```python
from build123d import *

# Parameters (mm, degrees)
F1_DEPTH      = 10
F3_DEPTH      = 10
F4_DEPTH      = 9
F5_DEPTH      = 9
F6_SIZE2      = 2.49999
F6_SIZE       = 1.49999
F7_R          = 0.8
F8_R          = 0.8
F9_R          = 0.8
F10_T1_DEPTH  = 10
F10_T4_ANGLE  = 88.2100893918
F10_T6_ANGLE  = 88.2100893918
F10_T8_ANGLE  = 88.2100893918
F10_T10_ANGLE = 88.2100893918


# Not quite as in the source:
# - a fillet or chamfer that OpenCascade refuses, or shapes differently, is made with other operations: its cross-section is extruded or revolved along the edge and cut away or added
# - a fillet or chamfer is up to 0.001 mm smaller than in the source, because OpenCascade refuses the exact size


with BuildPart() as f1:
    # F0 (on Top) → F1 (new body)
    with BuildSketch(Plane.XY):
        Polygon((27.5, 0), (-27.5, 0), (-28, 16), (-30.9985362283, 15.9062957429), (-30.4077144863, -3), (30.4077144863, -3), (30.9985362283, 15.9062957429), (28, 16), align=None)
        Polygon((-30.9985362283, 15.9062957429), (-28, 16), (-24.0019516957, 16.1249390095), (-24.0956559528, 19.1234752378), (-35.0902887897, 18.7798929616), (-34.9965845326, 15.7813567334), align=None)
        Polygon((24.0019516957, 16.1249390095), (28, 16), (30.9985362283, 15.9062957429), (34.9965845326, 15.7813567334), (34.9965845326, 18.7813567334), (24.0019516957, 19.1249390095), align=None)
    extrude(amount=F1_DEPTH)

    # F2 (on Right) → F3 (join, symmetric)
    with BuildSketch(Plane.YZ):
        Polygon((-3, 16), (-3, 10), (-0.5, 10), (-0.5, 20), (-3, 20), align=None)
    extrude(amount=F3_DEPTH, both=True)

    # F2 (on Right) → F4 (join, symmetric)
    with BuildSketch(Plane.YZ):
        Polygon((-3, 1.5), (-3, 10), (-3, 16), (-5, 16), (-5, 1.5), align=None)
    extrude(amount=F4_DEPTH, both=True)

    # F2 (on Right) → F5 (join, symmetric)
    with BuildSketch(Plane.YZ):
        Polygon((-5, 0), (-5, 1.5), (-5, 16), (-5, 18), (-7.5, 18), (-7.5, 0), align=None)
    extrude(amount=F5_DEPTH, both=True)

    # F6 (size 1.5 and 2.5 in the source; OpenCascade refuses exactly that, so slightly less here)
    f6_edges = [f1.edges().sort_by_distance(p)[0] for p in [
        (0, -7.5, 18),
        (-9, -7.5, 9),
        (9, -7.5, 9),
    ]]
    f6_side = f1.faces().sort_by_distance((0, -7.5, 9))[0]
    chamfer(f6_edges, length=F6_SIZE, length2=F6_SIZE2, reference=f6_side)

    # F7
    f7_edges = [f1.edges().sort_by_distance(p)[0] for p in [
        (27.75, 8, 0),
        (0, 0, 0),
        (-27.75, 8, 0),
        (-26.000976, 16.06247, 0),
        (-24.048804, 17.624207, 0),
        (-29.592972, 18.951684, 0),
        (-35.043437, 17.280625, 0),
        (-32.99756, 15.843826, 0),
        (-30.703125, 6.453148, 0),
        (0, -3, 0),
        (30.703125, 6.453148, 0),
        (32.99756, 15.843826, 0),
        (34.996585, 17.281357, 0),
        (29.499268, 18.953148, 0),
        (24.001952, 17.624939, 0),
        (26.000976, 16.06247, 0),
    ]]
    fillet(f7_edges, radius=F7_R)

    # F8
    f8_edges = [f1.edges().sort_by_distance(p)[0] for p in [
        (-29.592972, 18.951684, 10),
        (-35.043437, 17.280625, 10),
        (-32.99756, 15.843826, 10),
        (-26.000976, 16.06247, 10),
        (-24.048804, 17.624207, 10),
        (-27.75, 8, 10),
        (-30.703125, 6.453148, 10),
        (-20.203857, -3, 10),
        (20.203857, -3, 10),
        (30.703125, 6.453148, 10),
        (32.99756, 15.843826, 10),
        (34.996585, 17.281357, 10),
        (29.499268, 18.953148, 10),
        (24.001952, 17.624939, 10),
        (26.000976, 16.06247, 10),
        (27.75, 8, 10),
    ]]
    fillet(f8_edges, radius=F8_R)

    # F9
    f9_edges = [f1.edges().sort_by_distance(p)[0] for p in [
        (0, -0.5, 20),
        (-10, -0.5, 15),
        (10, -0.5, 15),
        (10, -1.75, 20),
        (-10, -1.75, 20),
    ]]
    fillet(f9_edges, radius=F9_R)

    # F10: fillet of radius 2 on 2 edges, made by hand

    # F10_s2 → F10_t1 (cut)
    with BuildSketch(Plane.XY):
        with BuildLine():
            ThreePointArc((-28.4692381621, -3), (-29.861190207, -2.4361300445), (-30.4682623143, -1.0624695048))
            Line((-30.4682623143, -1.0624695048), (-30.4077144863, -3))
            Line((-30.4077144863, -3), (-28.4692381621, -3))
        make_face()
        with BuildLine():
            ThreePointArc((28.4692381621, -3), (29.861190207, -2.4361300445), (30.4682623143, -1.0624695048))
            Line((30.4682623143, -1.0624695048), (30.4077144863, -3))
            Line((30.4077144863, -3), (28.4692381621, -3))
        make_face()
    extrude(amount=F10_T1_DEPTH, mode=Mode.SUBTRACT)

    # F10_s3 → F10_t4 (revolve, cut)
    with BuildSketch(Plane(origin=(-0.0034446457, -0.1102286623, 0), x_dir=(0, 0, 1), z_dir=(0.0312347524, 0.9995120761, 0))):
        with BuildLine():
            ThreePointArc((0, 29.6865820924), (0.2343145751, 30.2522675173), (0.8, 30.4865820924))
            Line((0.8, 30.4865820924), (0, 30.4865820924))
            Line((0, 30.4865820924), (0, 29.6865820924))
        make_face()
    revolve(axis=Axis((28.4692381621, -1, 0), (0, 0, -1)), revolution_arc=F10_T4_ANGLE, mode=Mode.SUBTRACT)

    # F10_s5 → F10_t6 (revolve, cut)
    with BuildSketch(Plane.YZ.offset(28.4692381621)):
        with BuildLine():
            ThreePointArc((-2.2, 10), (-2.7656854249, 9.7656854249), (-3, 9.2))
            Line((-3, 9.2), (-3, 10))
            Line((-3, 10), (-2.2, 10))
        make_face()
    revolve(axis=Axis((28.4692381621, -1, 10), (0, 0, 1)), revolution_arc=F10_T6_ANGLE, mode=Mode.SUBTRACT)

    # F10_s7 → F10_t8 (revolve, cut)
    with BuildSketch(Plane.YZ.offset(-28.4692381621)):
        with BuildLine():
            ThreePointArc((-2.2, 0), (-2.7656854249, 0.2343145751), (-3, 0.8))
            Line((-3, 0.8), (-3, 0))
            Line((-3, 0), (-2.2, 0))
        make_face()
    revolve(axis=Axis((-28.4692381621, -1, 0), (0, 0, -1)), revolution_arc=F10_T8_ANGLE, mode=Mode.SUBTRACT)

    # F10_s9 → F10_t10 (revolve, cut)
    with BuildSketch(Plane(origin=(0.0034446457, -0.1102286623, 0), x_dir=(0, 0, 1), z_dir=(-0.0312347524, 0.9995120761, 0))):
        with BuildLine():
            ThreePointArc((10, -29.6865820924), (9.7656854249, -30.2522675173), (9.2, -30.4865820924))
            Line((9.2, -30.4865820924), (10, -30.4865820924))
            Line((10, -30.4865820924), (10, -29.6865820924))
        make_face()
    revolve(axis=Axis((-28.4692381621, -1, 10), (0, 0, 1)), revolution_arc=F10_T10_ANGLE, mode=Mode.SUBTRACT)


solid = f1.part
```
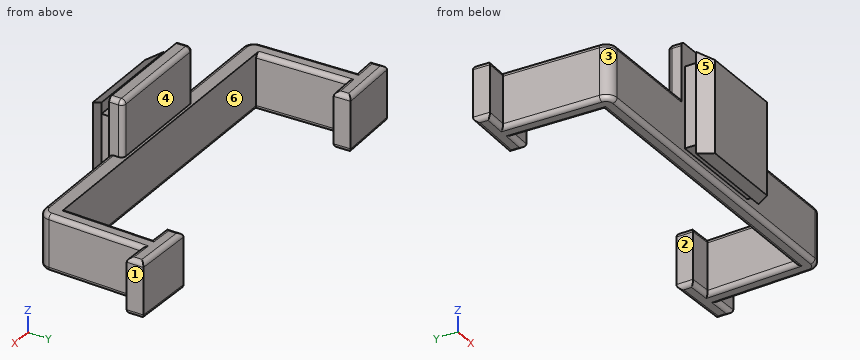
Can you work these out from the model? Positions are in its coordinate system, mm. Face numbers are marked on the shaded views. A direction names the side the tool comes from. Round coordinates to 2 decimals unless told otherwise and drop trailing zeros. Loops run counter-clockwise (first coordinate to the right, second up) from the corner with the lowest first, then second, coordinate; pieces in that order, holes last. Notation, with made-up numbers: M 73.25,64.5 L 117.25,64.5 A26 cw 117.25,78.5 Z; hole C 76,25.5 d1. An arc over 180 degrees is marked long. Answer as a JSON object with one key per item and string values. Group by question number.
Q1. We'd pull the mould along X, two halves only. Please class the marked faces 1, 2 and 3: +X half, -X half, draft (parallel to the pull), parting line (faces both ways), or undercut.
Q2. Imagine slicing it at B-B, the plane z = 11.75. Please give me the cut outline in (x, y), then the cut area to 3 significant figures.
Q3. Will these pins go through, and if not, where does the flat tip stop? pin 1 (1.9 mm diameter, centred on y = -1.5, z = 12, fed in from -X); pin 2 (12 mm diameter, centred on y = 2, z = 15, fed in from +X); pin 3 (1 mm diameter, centred on y = 6.5, z = 8, fed in from -X); pin 4 (3 mm diameter, centred on y = 7.5, z = 12.5, fed in from +X).
Q4. Imagine slicing it at A-A, the plane x = 22.5. Please give me the cut outline in (y, z), then the cut area to 3 significant figures.
Q5. Imagine slicing it at C-C, the plane z = 3.25. Please give me the cut outline in (x, y), then the cut area to 3 significant figures.
Q6. Please list where these lines run through material, in increasing order: L1, parallel to Z at x = -30, y = 13.75; L2, parallel to X at y = 14.25, z = 3; L3, parallel to Y at x = 6.5, z = 6.75.
Q7. On a 3-axis mill with a long thin cutter (end or side, diameter ignored), from which of +Z, -Z, +X, -X, +Y, -Y can I reach the whole of each face in a straight line? I mean the marked faces 4, 5 and 6. Say none if no direction works.
Findings:
{
 "1": {"face 1": "+X half", "face 2": "undercut", "face 3": "-X half"},
 "2": {"outline": "M -10,-3 L -9,-3 L -9,-5 L -7.5,-7.5 L 7.5,-7.5 L 9,-5 L 9,-3 L 10,-3 L 10,-1.3 A0.8 ccw 9.2,-0.5 L -9.2,-0.5 A0.8 ccw -10,-1.3 Z", "area": "127 mm2"},
 "3": {"pin 1": "stops at x = -10", "pin 2": "stops at x = 30.62", "pin 3": "stops at x = -30.72", "pin 4": "passes through"},
 "4": {"outline": "M -3,0.8 A0.8 ccw -2.2,0 L -0.8,0 A0.8 ccw 0,0.8 L 0,10 L -2.2,10 A0.8 ccw -3,9.2 Z", "area": "29.6 mm2"},
 "5": {"outline": "M -35.09,18.78 L -35,15.78 L -31,15.91 L -30.47,-1.06 A2 ccw -28.47,-3 L -9,-3 L -9,-5 L -7.5,-7.5 L 7.5,-7.5 L 9,-5 L 9,-3 L 28.47,-3 A2 ccw 30.47,-1.06 L 31,15.91 L 35,15.78 L 35,18.78 L 24,19.12 L 24,16.12 L 28,16 L 27.5,0 L -27.5,0 L -28,16 L -24,16.12 L -24.1,19.12 Z", "area": "420 mm2"},
 "6": {"L1": "z = 0 to 10", "L2": "x = -30.95 to -27.95, 27.95 to 30.95", "L3": "y = -7.5 to 0"},
 "7": {"face 4": "+Z, +X, -X, +Y", "face 5": "+Z, -Z, -X, -Y", "face 6": "+Z, -Z"}
}
